Verification items for the finished model (mm, model axes). Face numbers are marked on the shaded views. A direction names the side the tool comes from. Coordinates: 2 decimals unless noted, no trailing zeros. Loops run counter-clockwise (first coordinate to the right, second up) from the corner with the lowest first, then second, coordinate; pieces in that order, holes last. Notation, with made-up numbers: (-23.75, 15) -> (-2.75, 15) arc R28 ccw to (-2.75, 48) -> close; hole circle Ø5 at (-1.75, 22.25). An arc over 180 degrees is marked (long way). Write item = value, one per line.
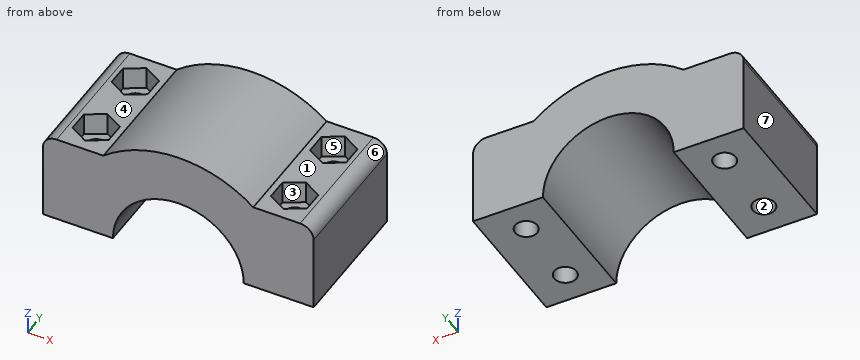
Autodesk Inventor part; units mm, degrees
ref_plane "YZ Plane" through (0, 0, 0) normal (1, 0, 0) x (0, 1, 0)
ref_plane "XZ Plane" through (0, 0, 0) normal (0, 1, 0) x (-1, 0, 0)
ref_plane "XY Plane" through (0, 0, 0) normal (0, 0, 1) x (1, 0, 0)
sketch "Schizzo1" plane through (0, 0, 0) normal (0, 0, 1) x (1, 0, 0)
  line L0 (-30, -15) -> (30, -15)
  line L1 (30, -15) -> (30, 15)
  line L2 (30, 15) -> (-30, 15)
  line L3 (-30, 15) -> (-30, -15)
  line L4 (-30, -15) -> (30, 15) construction
  line L5 (30, -15) -> (-30, 15) construction
  point P0 (0, 0)
  point P1 (0, 0)
  dimension "d27" = 30
  dimension "d28" = 60
extrude "Estrusione1" add sketch "Schizzo1" against normal blind 20
sketch "Schizzo2" plane through (-25, 15, 0) normal (0, 1, 0) x (1, 0, 0)
  line L0 (55, 20) -> (-5, 20)
  circle A0 centre (25, 20) radius 14.5
  point P0 (25, 0)
  dimension "d60" = 29
  dimension "d61" = 20
extrude "Estrusione2" cut sketch "Schizzo2" against normal blind 30
sketch "Schizzo6" plane through (0, 0, 0) normal (0, 0, 1) x (1, 0, 0)
  line L0 (0, 15) -> (0, 8)
  line L1 (0, 8) -> (-22, 8)
  line L2 (-22, 8) -> (-22, -8)
  line L3 (0, 8) -> (22, 8)
  line L4 (0, 8) -> (22, 8) construction
  line L5 (22, 8) -> (22, -8)
  point P0 (0, 0)
  dimension "d29" = 7
  dimension "d30" = 22
  dimension "d31" = 90
  dimension "d32" = 16
  dimension "d33" = 90
  dimension "d34" = 22
  dimension "d36" = 16
  dimension "d37" = 90
hole "Foro3" at (-22, 8, 0) at (-22, -8, 0) at (22, -8, 0) at (22, 8, 0) direction (0, 0, -1) diameter 4.9 end through all
sketch "Schizzo7" plane through (0, 0, 0) normal (0, 0, 1) x (1, 0, 0)
  line L0 (-14.5, 15) -> (14.5, 15)
  line L1 (0, 15) -> (0, 8)
  line L2 (0, 8) -> (-22, 8)
  line L3 (-22, 8) -> (-22, -8)
  line L4 (0, 8) -> (22, 8)
  line L5 (0, 8) -> (22, 8) construction
  line L6 (22, 8) -> (22, -8)
  circle A0 centre (-22, -8) radius 4
  circle A1 centre (22, 8) radius 4
  circle A2 centre (22, -8) radius 4
  circle A3 centre (-22, 8) radius 4
  line L7 (-18, 5.6906) -> (-22, 3.3812)
  line L8 (-22, 3.3812) -> (-26, 5.6906)
  line L9 (-26, 5.6906) -> (-26, 10.3094)
  line L10 (-26, 10.3094) -> (-22, 12.6188)
  line L11 (-22, 12.6188) -> (-18, 10.3094)
  line L12 (-18, 10.3094) -> (-18, 5.6906)
  line L13 (-18, -10.3094) -> (-22, -12.6188)
  line L14 (-22, -12.6188) -> (-26, -10.3094)
  line L15 (-26, -10.3094) -> (-26, -5.6906)
  line L16 (-26, -5.6906) -> (-22, -3.3812)
  line L17 (-22, -3.3812) -> (-18, -5.6906)
  line L18 (-18, -5.6906) -> (-18, -10.3094)
  line L19 (26, -10.3094) -> (22, -12.6188)
  line L20 (22, -12.6188) -> (18, -10.3094)
  line L21 (18, -10.3094) -> (18, -5.6906)
  line L22 (18, -5.6906) -> (22, -3.3812)
  line L23 (22, -3.3812) -> (26, -5.6906)
  line L24 (26, -5.6906) -> (26, -10.3094)
  line L25 (26, 5.6906) -> (22, 3.3812)
  line L26 (22, 3.3812) -> (18, 5.6906)
  line L27 (18, 5.6906) -> (18, 10.3094)
  line L28 (18, 10.3094) -> (22, 12.6188)
  line L29 (22, 12.6188) -> (26, 10.3094)
  line L30 (26, 10.3094) -> (26, 5.6906)
  point P0 (0, 0)
  point P1 (0, 0)
  point P2 (-18, 8)
  point P3 (-18, -8)
  point P4 (26, -8)
  point P5 (26, 8)
  point P6 (-24, -11.4641)
  point P7 (-20, -11.4641)
  point P8 (-26, -8)
  point P9 (-24, -4.5359)
  point P10 (-20, -4.5359)
  dimension "d54" = 8
  dimension "d55" = 8
  dimension "d56" = 8
  dimension "d69" = 8
  dimension "d45" = 7
  dimension "d46" = 22
  dimension "d47" = 90
  dimension "d48" = 16
  dimension "d49" = 90
  dimension "d50" = 22
  dimension "d51" = 16
extrude "Estrusione4" cut sketch "Schizzo7" against normal blind 5
fillet "Raccordo1" radius 3 1 edges at (30, 0, 0)
fillet "Raccordo2" radius 3 1 edges at (-30, 0, 0)
sketch "Schizzo9" plane through (0, 15, -20) normal (0, 1, 0) x (1, 0, 0)
  circle A0 centre (0, 0) radius 26
  line L0 (27, -20) -> (-27, -20)
  line L1 (16.6132, -20) -> (-16.6132, -20)
  point P0 (0, -20)
  dimension "d66" = 52
extrude "Estrusione5" add sketch "Schizzo9" against normal blind 30 contours L0 A0 picked at (-3.8639, -21.091)
properties part number "3_Connettore_inf_INF" material "PLA(Stampato)(D0,646)"
1) Release check for a two-part mould opening along X. For the marked faces 4, 5, 6 and 7 record: pulls with the +X half, pulls with the -X half, needs draft (parallel to the pull), parting line crosses it, or undercut.
Ans:
face_4 = needs draft
face_5 = undercut
face_6 = pulls with the +X half
face_7 = pulls with the -X half
2) Sectioned sample at B-B, the plane x = 23. Record the cut outline in (y, z), plus the area to 3 significant figures.
Ans:
outline = (-15, -20) -> (-10.24, -20) -> (-10.24, -5) -> (-12.04, -5) -> (-12.04, 0) -> (-15, 0) -> close; (-5.76, -20) -> (5.76, -20) -> (5.76, -5) -> (3.96, -5) -> (3.96, 0) -> (-3.96, 0) -> (-3.96, -5) -> (-5.76, -5) -> close; (10.24, -20) -> (15, -20) -> (15, 0) -> (12.04, 0) -> (12.04, -5) -> (10.24, -5) -> close
area = 385 mm2
3) Depth check by flat-ended pin: pin 1 Ø6.5 at (x, y) = (22, 8) entering from +Z; pin 2 Ø1.5 at (x, y) = (11.5, 3) entering from -Z; pin 3 Ø2.5 at (y, z) = (8.5, -1.5) entering from -X; pin 4 Ø2.5 at (x, y) = (-21.5, 8) entering from +Z. Enter the tip coordinate at first touch or a pass-through.
Ans:
pin_1 = -5
pin_2 = -12.24
pin_3 = -29.99
pin_4 = through
4) Material ranges on line 1 (Y direction, x = 22, z = -8.75); line 2 (Y direction, x = 23, z = -13.5); line 3 (X direction, y = 5.5, z = -0.5), recorded low to high.
Ans:
line_1 = -15 to -10.45, -5.55 to 5.55, 10.45 to 15
line_2 = -15 to -10.24, -5.76 to 5.76, 10.24 to 15
line_3 = -28.66 to -25.67, -18.33 to 18.33, 25.67 to 28.66
5) Sectioned sample at D-D, the plane z = -6.5. Record the cut outline in (x, y).
Ans:
outline = (-30, -15) -> (-5.29, -15) -> (-5.29, 15) -> (-30, 15) -> close; (5.29, -15) -> (30, -15) -> (30, 15) -> (5.29, 15) -> close; hole circle Ø4.9 at (-22, -8); hole circle Ø4.9 at (-22, 8); hole circle Ø4.9 at (22, -8); hole circle Ø4.9 at (22, 8)
6) Sectioned sample at C-C, the plane y = 8. Record the cut outline in (x, z), plus the area to 3 significant figures.
Ans:
outline = (-30, -20) -> (-24.45, -20) -> (-24.45, -5) -> (-26, -5) -> (-26, 0) -> (-27, 0) arc R3 ccw to (-30, -3) -> close; (-19.55, -20) -> (-14.5, -20) arc R14.5 cw to (14.5, -20) -> (19.55, -20) -> (19.55, -5) -> (18, -5) -> (18, 0) -> (16.61, 0) arc R26 ccw to (-16.61, 0) -> (-18, 0) -> (-18, -5) -> (-19.55, -5) -> close; (24.45, -20) -> (30, -20) -> (30, -3) arc R3 ccw to (27, 0) -> (26, 0) -> (26, -5) -> (24.45, -5) -> close
area = 775 mm2
7) Tool access check on the marked faces 1, 2 and 3. Record the directions out of +Z, -Z, +X, -X, +Y, -Y that give a thin tool (end or side, any length) a straight path to the whole face; none if there is none.
Ans:
face_1 = +Z, +X, +Y, -Y
face_2 = +Z, -Z
face_3 = +Z
8) Sectioned sample at A-A, the plane z = -12.5. Record the cut outline in (x, y), plus the area to 3 significant figures.
Ans:
outline = (-30, -15) -> (-12.41, -15) -> (-12.41, 15) -> (-30, 15) -> close; (12.41, -15) -> (30, -15) -> (30, 15) -> (12.41, 15) -> close; hole circle Ø4.9 at (-22, -8); hole circle Ø4.9 at (-22, 8); hole circle Ø4.9 at (22, -8); hole circle Ø4.9 at (22, 8)
area = 980 mm2
